Autodesk Inventor part; units mm, degrees
ref_plane "YZ Plane" through (0, 0, 0) normal (1, 0, 0) x (0, 1, 0)
ref_plane "XZ Plane" through (0, 0, 0) normal (0, 1, 0) x (-1, 0, 0)
ref_plane "XY Plane" through (0, 0, 0) normal (0, 0, 1) x (1, 0, 0)
sketch "Sketch1" plane through (0, 0, 0) normal (0, 0, 1) x (1, 0, 0)
  line L0 (0, 0) -> (14, 0)
  line L1 (14, 0) -> (14, 8.5)
  line L2 (14, 8.5) -> (0, 8.5)
  line L3 (0, 8.5) -> (0, 0)
  dimension "d0" = 14
  dimension "d1" = 8.5
extrude "Extrusion1" add sketch "Sketch1" along normal blind 2
sketch "Sketch2" plane through (14, 0, 0) normal (1, 0, 0) x (0, 0, -1)
  line L0 (-2, 8.5) -> (-2, 0)
  line L1 (0, 0) -> (-2, 0)
  line L2 (0, 8.5) -> (-2, 8.5)
  arc A0 (-2, 8.5) -> (-2, 0) centre (-2, 4.25) ccw
  line L3 (-2, 8.5) -> (-2, 0)
extrude "Extrusion2" add sketch "Sketch2" against normal blind 14
chamfer "Chamfer1" distance 2 angle 10 1 edges at (7, 0, 0) measured on face at (4.6667, 0, 0.6667)
chamfer "Chamfer2" distance 2 angle 10 1 edges at (7, 8.5, 0) measured on face at (9.3333, 8.5, 0.6667)
sketch "Sketch3" plane through (0, 0, 0) normal (0, 0, -1) x (-1, 0, 0)
  line L0 (-14, 8.1473) -> (0, 8.1473)
  line L1 (-14, 0.3527) -> (-14, 8.1473)
  line L2 (0, 0.3527) -> (-14, 0.3527)
  line L3 (0, 8.1473) -> (0, 0.3527)
  point P0 (0, 0)
hole "Hole1" at (7, 4.2527, 0) direction (0, 0, 1) diameter 4 end through all
hole "Hole2" at (7, 4.2527, 0) direction (0, 0, 1) diameter 8.1 depth 3.5
properties part number "cam pivot"
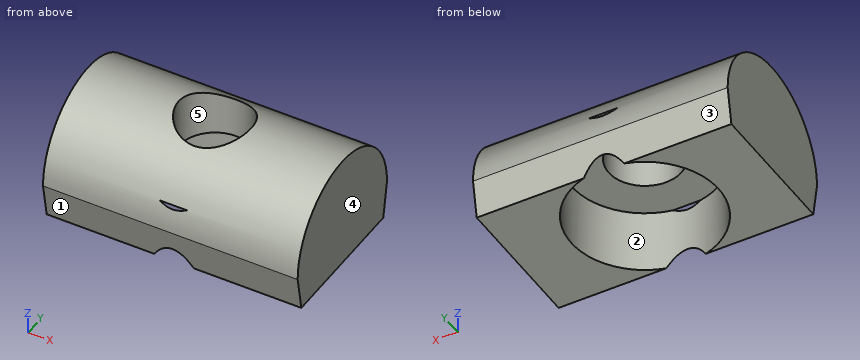
Can you work these out from the model? Positions are in its coordinate system, mm. Face numbers are marked on the shaded views. A direction names the side the tool comes from. Coordinates: 2 decimals unless noted, no trailing zeros. Order: outer loops, then holes, each group sorted by start corner. A loop starts at its lowest first (then second) coordinate and runs counter-clockwise, first axis right, second up.
1. If we section it at A-A (y = 4.25): Please give me the cut outline in (x, z).
2. If we section it at C-C (y = 5.5): Please give me the cut outline in (x, z), then the cut area to 3 significant figures.
3. I'm going to push flat-ended pins straight in: pin 1 (1 mm diameter, centred on x = 9.5, y = 5, fed in from -Z); pin 2 (1 mm diameter, centred on x = 2, z = 3.5, fed in from +Y); pin 3 (3 mm diameter, centred on x = 11.5, z = 4, fed in from +Y). Where does each tip first touch, or does it pass through?
4. For the marked faces 1 and 2, which set-ups out of +Z, -Z, +X, -X, +Y, -Y let a thin tool reach every point of the face, with its end or its side?
5. If we section it at D-D (x = 7): Give the number of separate pieces and of enclosed holes in the cut face, then the cut area to 3 significant figures.
6. I need wall thicknesses on line 1 (X direction, y = 2.5, z = 1.75); line 2 (X direction, y = 3.75, z = 2.5); line 3 (Y direction, x = 7, z = 4.9). Which ranges of each line are inside material? Lowest first, please.
7. Thinking about a two-plate mould opening in Y: for the marked faces 3, 4 and 5, which applies, +Y half, -Y half, draft (parallel to the pull), parting line (faces both ways), or undercut?
Entries:
1. outline: (0, 0) - (2.95, 0) - (2.95, 3.5) - (5, 3.5) - (5, 6.25) - (0, 6.25) - close; (9, 3.5) - (11.05, 3.5) - (11.05, 0) - (14, 0) - (14, 6.25) - (9, 6.25) - close
2. outline: (0, 0) - (3.15, 0) - (3.15, 3.5) - (5.44, 3.5) - (5.44, 6.06) - (0, 6.06) - close; (8.56, 3.5) - (10.85, 3.5) - (10.85, 0) - (14, 0) - (14, 6.06) - (8.56, 6.06) - close
2. area: 49.9 mm2
3. pin 1: stops at z = 3.5
3. pin 2: stops at y = 8.38
3. pin 3: stops at y = 8.47
4. face 1: -Z, +X, -X, -Y
4. face 2: -Z
5. separate pieces: 4
5. enclosed holes: 0
5. area: 6.12 mm2
6. line 1: x = 0 to 3.35, 10.65 to 14
6. line 2: x = 0 to 2.98, 11.02 to 14
6. line 3: y = 1.14 to 2.25, 6.25 to 7.36
7. face 3: +Y half
7. face 4: draft
7. face 5: undercut
